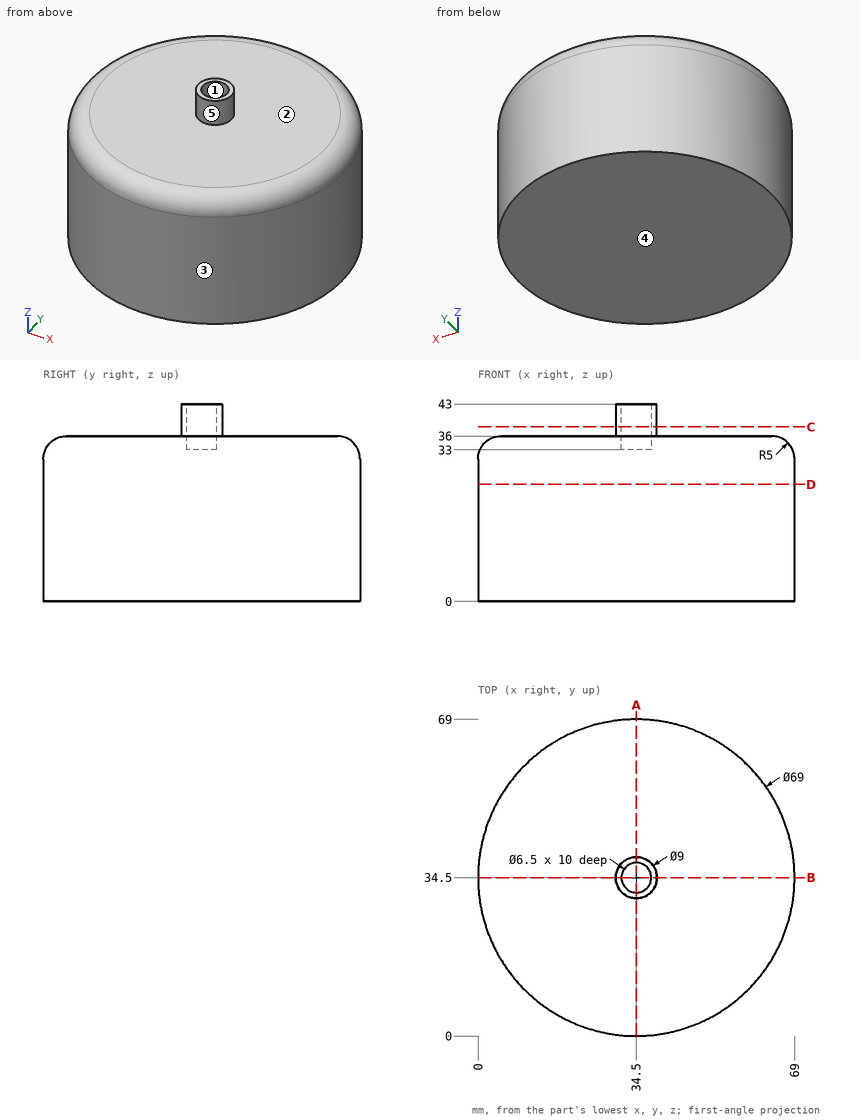
Drawing for the job (mm, zero at the part's lowest x, y, z). A direction names the side the tool comes from. Round coordinates to 2 decimals unless told otherwise and drop trailing zeros. Write each loop counter-clockwise with the first axis right and the second up, starting at its lowest first coordinate (ties: lowest second). Pieces come first, ordered by that corner, then holes. Notation, with made-up numbers: M 1,14 L 5,14 A26 cw 5,30 Z; hole C 25.5,48.25 d9. An arc over 180 degrees is marked long. One line per question, with ' | ' between items.
1. Cut at C-C on z = 38. Write the cut outline in (x, y).
Working result:
outline: C 34.5,34.5 d9; hole C 34.5,34.5 d6.5
2. Cut at D-D on z = 25.5. Write the cut outline in (x, y), and give its area (3 significant figures).
Working result:
outline: C 34.5,34.5 d69 | area: 3,740 mm2
3. Probe L1, parallel to Y at x = 34.5, z = 41.25; L2, parallel to Y at x = 37.5, z = 37.5; L3, parallel to Z at x = 46.5, y = 18.5. List the from-to ranges inside material, lowest first. Write a range as from..to.
Working result:
L1: 30..31.25, 37.75..39 | L2: 31.15..33.25, 35.75..37.85 | L3: 0..36
4. Which spindle directions (+Z, -Z, +X, -X, +Y, -Y) get a long thin tool onto all of the face, cutting with end or side? Do the marked faces 4 and 5. Say none if no direction does.
Working result:
face 4: -Z, +X, -X, +Y, -Y | face 5: +Z
5. Pin check, flat tips, straight feed: pin 1 Ø10 at (x, z) = (9, 28) entering from +Y; pin 2 Ø1 at (x, z) = (53, 6) entering from -Y; pin 3 Ø4 at (x, y) = (34.5, 34.5) entering from +Z. Stop position of each tip, or through.
Working result:
pin 1: y = 62.25 | pin 2: y = 5.07 | pin 3: z = 33
6. Mould opens along X. For the marked faces 1, 2 and 3 say: pulls with the +X half, pulls with the -X half, needs draft (parallel to the pull), parting line crosses it, or undercut.
Working result:
face 1: undercut | face 2: needs draft | face 3: parting line crosses it
7. Cut at A-A on x = 34.5. Write the cut outline in (y, z), and give its area (3 significant figures).
Working result:
outline: M 0,0 L 69,0 L 69,31 A5 ccw 64,36 L 39,36 L 39,43 L 37.75,43 L 37.75,33 L 31.25,33 L 31.25,43 L 30,43 L 30,36 L 5,36 A5 ccw 0,31 Z | area: 2,470 mm2
